```python
from build123d import *

# Parameters (mm, degrees)
F0_W     = 241.3
F0_H     = 76.2
F1_DEPTH = 60.325
F3_DEPTH = 76.201


with BuildPart() as f1:
    # F0 (on Top) → F1 (new body)
    with BuildSketch(Plane.XY):
        with Locations((120.65, 38.1)):
            Rectangle(F0_W, F0_H)
    extrude(amount=F1_DEPTH)

    # F2 (on Front) → F3 (cut, through all)
    with BuildSketch(Plane.XZ):
        with BuildLine():
            Line((65.0748, 52.3748), (0, 52.3748))
            Line((0, 52.3748), (0, 0))
            Line((0, 0), (88.9, 0))
            ThreePointArc((88.9, 0), (77.67468, 4.64968), (73.025, 15.875))
            Line((73.025, 15.875), (73.025, 44.4246))
            ThreePointArc((73.025, 44.4246), (70.69644, 50.04624), (65.0748, 52.3748))
        make_face()
        with BuildLine():
            Line((176.1998, 60.325), (65.1002, 60.325))
            ThreePointArc((65.1002, 60.325), (76.32552, 55.67532), (80.9752, 44.45))
            Line((80.9752, 44.45), (80.9752, 15.9004))
            ThreePointArc((80.9752, 15.9004), (83.30376, 10.27876), (88.9254, 7.9502))
            Line((88.9254, 7.9502), (152.44318, 7.9502))
            ThreePointArc((152.44318, 7.9502), (158.016327, 10.258673), (160.3248, 15.83182))
            Line((160.3248, 15.83182), (160.3248, 44.45))
            ThreePointArc((160.3248, 44.45), (164.97448, 55.67532), (176.1998, 60.325))
        make_face()
        with BuildLine():
            ThreePointArc((168.275, 15.875), (163.62532, 4.64968), (152.4, 0))
            Line((152.4, 0), (241.3, 0))
            Line((241.3, 0), (241.3, 52.3748))
            Line((241.3, 52.3748), (176.2252, 52.3748))
            ThreePointArc((176.2252, 52.3748), (170.60356, 50.04624), (168.275, 44.4246))
            Line((168.275, 44.4246), (168.275, 15.875))
        make_face()
    extrude(amount=-F3_DEPTH, mode=Mode.SUBTRACT)


solid = f1.part
```
The listing builds one solid part. Answer for the finished solid, in the listing's coordinates (mm). A direction names the side the tool comes from. Round coordinates to 2 decimals unless told otherwise and drop trailing zeros. Write each loop counter-clockwise with the first axis right and the second up, starting at its lowest first coordinate (ties: lowest second). Pieces come first, ordered by that corner, then holes. Notation, with made-up numbers: (-11, 69) -> (-2, 69) arc R32 ccw to (-2, 102) -> close; hole circle Ø6 at (77.5, -14.75). An arc over 180 degrees is marked (long way). Use CSV: the item, a comma, the result in double quotes. Start each with the question number.
(1) Consider L1, parallel to X at y = 18.5, z = 42 (3 decimals); L2, parallel to Z at x = 54.5, y = 16 (3 decimals); L3, parallel to Z at x = 105, y = 56.5. Determine where each line is inside the solid, lowest interval first. Write a range as from..to.
(2) Section B-B on y = 67.5 is taken. Give the vertices of the cut face in (x, z) (3 decimals).
(3) Section C-C on z = 47 is taken. Give the vertices of the cut face in (x, y), then the cut area to 3 significant figures.
(4) Section A-A on z = 20.5 is taken. Give the vertices of the cut face in (x, y) (3 decimals), then the cut area to 3 significant figures.
(5) Which of the six approach directions +Z, -Z, +X, -X, +Y, -Y give full straight-line access (tool end or side, diameter ignored) to faces 4 (the face through (209, 38, 52.375)), 5 (the face through (80.975, 38, 30)), 6 (the face through (33, 38, 52.375)), 7 (the face through (120, 39, 0))?
(6) Section D-D on x = 183 is taken. Give the vertices of the cut face in (y, z) (3 decimals), then the cut area to 3 significant figures.
(7) The mould has two halves that part along X. Classify faces 1 (the face through (32, 39, 60.325)), 2 (the face through (83.242, 37.567, 10.341)), 3 (the face through (241.3, 38, 56)): released by +X, released by -X, zero draft, split by the parting line, or undercut.
(8) Each of these flat-tipped pins is pushed along its axis until it touches: pin 1 (5 mm diameter, centred on x = 74, y = 21.5, fed in from -Z); pin 2 (2 mm diameter, centred on y = 16, z = 42.5, fed in from -X) (3 decimals); pin 3 (6 mm diameter, centred on x = 183, y = 13.5, fed in from -Z); pin 4 (5 mm diameter, centred on x = 155.5, z = 36, fed in from +Y). Where does it stop, or does it pass through?
A:
1,L1,"x = 73.025..80.975, 160.325..168.275"
1,L2,"z = 52.375..60.325"
1,L3,"z = 0..7.95"
2,outline,"(0, 52.375) -> (65.075, 52.375) arc R7.95 cw to (73.025, 44.425) -> (73.025, 15.875) arc R15.875 ccw to (88.9, 0) -> (152.4, 0) arc R15.875 ccw to (168.275, 15.875) -> (168.275, 44.425) arc R7.95 cw to (176.225, 52.375) -> (241.3, 52.375) -> (241.3, 60.325) -> (176.2, 60.325) arc R15.875 ccw to (160.325, 44.45) -> (160.325, 15.832) arc R7.882 cw to (152.443, 7.95) -> (88.925, 7.95) arc R7.95 cw to (80.975, 15.9) -> (80.975, 44.45) arc R15.875 ccw to (65.1, 60.325) -> (0, 60.325) -> close"
3,outline,"(72.6, 0) -> (80.77, 0) -> (80.77, 76.2) -> (72.6, 76.2) -> close; (160.53, 0) -> (168.7, 0) -> (168.7, 76.2) -> (160.53, 76.2) -> close"
3,area,"1,250 mm²"
4,outline,"(73.025, 0) -> (80.975, 0) -> (80.975, 76.2) -> (73.025, 76.2) -> close; (160.325, 0) -> (168.275, 0) -> (168.275, 76.2) -> (160.325, 76.2) -> close"
4,area,"1,210 mm²"
5,face 4,"-Z, +X, +Y, -Y"
5,face 5,"+Z, +Y, -Y"
5,face 6,"-Z, -X, +Y, -Y"
5,face 7,"-Z, +X, -X, +Y, -Y"
6,outline,"(0, 52.375) -> (76.2, 52.375) -> (76.2, 60.325) -> (0, 60.325) -> close"
6,area,"606 mm²"
7,face 1,"zero draft"
7,face 2,"undercut"
7,face 3,"released by +X"
8,pin 1,"stops at z = 5.96"
8,pin 2,"stops at x = 73.025"
8,pin 3,"stops at z = 52.37"
8,pin 4,"passes through"
